Read the model definition and answer for the solid it produces. Units are mm, in the model's axes. Face numbers are marked on the shaded views. A direction names the side the tool comes from. Coordinates: 2 decimals unless noted, no trailing zeros. Write each loop counter-clockwise with the first axis right and the second up, starting at its lowest first coordinate (ties: lowest second). Pieces come first, ordered by that corner, then holes. Notation, with made-up numbers: (-28.5, 8.25) - (7.5, 8.25) arc R25 cw to (7.5, 31.25) - close; hole circle Ø3 at (61, 29.25). An arc over 180 degrees is marked (long way). Use a Markdown table: item, result.
from build123d import *

# Parameters (mm, degrees)
F0_W     = 368.3
F0_H     = 50.8
F1_DEPTH = 19.05
F2_DEPTH = 50.8
F3_DEPTH = 25.4
F5_DEPTH = 444.501
F7_DEPTH = 50.801


with BuildPart() as f1:
    # F0 (on Right) → F1 (new body)
    with BuildSketch(Plane.YZ):
        Rectangle(F0_W, F0_H)
    extrude(amount=F1_DEPTH)

    # F2 (add): a face of the model
    f2_faces = [f1.faces().sort_by_distance(p)[0] for p in [
        (9.525, -184.15, 0),
    ]]
    extrude(f2_faces, amount=F2_DEPTH)

    # F3 (add): a face of the model
    f3_faces = [f1.faces().sort_by_distance(p)[0] for p in [
        (9.525, 184.15, 0),
    ]]
    extrude(f3_faces, amount=F3_DEPTH)

    # F4 (on face) → F5 (cut, through all)
    with BuildSketch(Plane(origin=(0, 209.55, 0), x_dir=(-1, 0, 0), z_dir=(0, 1, 0))):
        Polygon((-6.35, 0), (-6.35, -25.4), (-6.35, -26.9535556436), (8.1521905959, -26.9535556436), (8.1521905959, 0), align=None)
    extrude(amount=-F5_DEPTH, mode=Mode.SUBTRACT)

    # F6 (on face) → F7 (cut, through all)
    with BuildSketch(Plane.XY.offset(25.4)):
        Polygon((0, 190.5), (19.05, 209.55), (19.2840322852, 224.0246832371), (-11.843809858, 224.0246832371), (-11.843809858, 190.5), align=None)
        Polygon((19.05, -242.6750212908), (19.05, -234.95), (0, -215.9), (-3.5010655411, -215.9), (-3.5010655411, -242.6750212908), align=None)
    extrude(amount=-F7_DEPTH, mode=Mode.SUBTRACT)


solid = f1.part
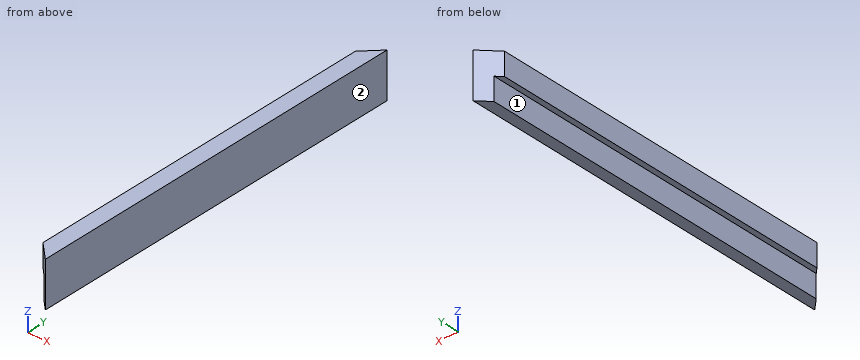
(1) Each of these flat-tipped pins is pushed along its axis until it touches: P1, Ø2, axis at x = 6, z = -8.5, coming from the +Y side; P2, Ø7.5, axis at y = 55, z = -18, coming from the -X side; P3, Ø5, axis at x = 13, z = -13.5, coming from the +Y side. Where does it stop, or does it pass through?
Report:
| item | result |
|---|---|
| P1 | stops at y = 197.5 |
| P2 | stops at x = 6.35 |
| P3 | stops at y = 206 |
(2) A cutting plane is placed at C-C, the plane z = 19.5. Write down the section's boundary in (x, y), and give its area (3 significant figures).
Report:
| item | result |
|---|---|
| outline | (0, -215.9) - (19.05, -234.95) - (19.05, 209.55) - (0, 190.5) - close |
| area | 8,100 mm² |
(3) For the marked faces 1 and 2, determine the directions among +Z, -Z, +X, -X, +Y, -Y from which every point of the face is accessible in a straight line to the end or side of a thin tool.
Report:
| item | result |
|---|---|
| face 1 | -Z, -X, +Y, -Y |
| face 2 | +Z, -Z, +X, +Y, -Y |
(4) A cutting plane is placed at B-B, the plane y = 120.5. Write down the section's boundary in (x, z), and give its area (3 significant figures).
Report:
| item | result |
|---|---|
| outline | (0, 0) - (6.35, 0) - (6.35, -25.4) - (19.05, -25.4) - (19.05, 25.4) - (0, 25.4) - close |
| area | 806 mm² |
(5) A cutting plane is placed at A-A, the plane x = 12. Write down the section's boundary in (y, z), and give its area (3 significant figures).
Report:
| item | result |
|---|---|
| outline | (-227.9, -25.4) - (202.5, -25.4) - (202.5, 25.4) - (-227.9, 25.4) - close |
| area | 21,900 mm² |
(6) Straight lines are drawn through the part: L1, parallel to Z at x = 3, y = 20.5; L2, parallel to X at y = 19, z = -23; L3, parallel to Y at x = 9.25, z = -20. For each, find the intervals that lie inside material, in ascending order.
Report:
| item | result |
|---|---|
| L1 | z = 0 to 25.4 |
| L2 | x = 6.35 to 19.05 |
| L3 | y = -225.15 to 199.75 |
